```python
from build123d import *

# Parameters (mm, degrees)
F0_R     = 63.5
F1_DEPTH = 127
F2_R     = 25.4
F2_R_2   = 24.093414
F3_DEPTH = 127


with BuildPart() as f1:
    # F0 (on Front) → F1 (new body)
    with BuildSketch(Plane.XZ):
        with Locations((-63.626207, 65.614522)):
            Circle(F0_R)
    extrude(amount=F1_DEPTH)

    # F2 (on face) → F3 (join)
    with BuildSketch(Plane(origin=(0, 0, 0), x_dir=(-1, 0, 0), z_dir=(0, 1, 0))):
        with Locations((61.020497, 71.783684)):
            Circle(F2_R)
        with Locations((61.020497, 71.783684)):
            Circle(F2_R_2, mode=Mode.SUBTRACT)
    extrude(amount=F3_DEPTH)


solid = f1.part
```
CAD build for the part. Positions are in the model's coordinates, mm. A direction names the side the tool comes from. Round coordinates to 2 decimals unless told otherwise and drop trailing zeros. Order: outer loops, then holes, each group sorted by start corner. A loop starts at its lowest first (then second) coordinate and runs counter-clockwise, first axis right, second up.
Q1. Wall check: L1, parallel to Y at x = -28, z = 102.5; L2, parallel to X at y = 62.5, z = 86; L3, parallel to X at y = 71, z = 58.5. Give the ranges that are in metal, low to high.
Q2. Drop flat-ended pins along their axis: pin 1 (1.5 mm diameter, centred on x = -108, z = 104, fed in from +Y); pin 2 (1 mm diameter, centred on y = -97.5, z = 19.5, fed in from -X); pin 3 (6 mm diameter, centred on y = -47.5, z = 48, fed in from -X). Give the stop position or say it passes through.
Q3. Two-plate mould, pull along X, no slides. Class faces 1 (the flat face through (-79, 0, 52)), 2 (the cylindrical face through (-72.14, 62.61, 50.41)), 3 (the cylindrical face through (-77.392, -62.611, 3.625)): pulls with the +X half, pulls with the -X half, needs draft (parallel to the pull), parting line crosses it, or undercut.
Q4. Slice it at B-B (x = -100). Write the cut outline in (y, z), and give its area (3 significant figures).
Q5. Slice it at D-D (z = 54.5). Write the cut outline in (x, y), and give its area (3 significant figures).
Q6. Slice it at C-C (y = 69.5). Write the cut outline in (x, z).
Q7. Which spindle directions (+Z, -Z, +X, -X, +Y, -Y) get a long thin tool onto all of the face, cutting with end or side? Do faces 4 (the flat face through (-65, -127, 67)), 5 (the cylindrical face through (-40.864, 62.611, 56.328)). Say none if no direction does.
Q8. Slice it at A-A (z = 91). Write the cut outline in (x, y).
Results below:
1. L1: y = -127 to 0
1. L2: x = -82.07 to -80.47, -41.57 to -39.97
1. L3: x = -82.67 to -81.12, -40.92 to -39.37
2. pin 1: stops at y = 0
2. pin 2: stops at x = -107.8
2. pin 3: stops at x = -125.42
3. face 1: needs draft
3. face 2: undercut
3. face 3: parting line crosses it
4. outline: (-127, 13.56) - (0, 13.56) - (0, 117.66) - (-127, 117.66) - close
4. area: 13,200 mm2
5. outline: (-126.15, -127) - (-1.11, -127) - (-1.11, 0) - (-42.41, 0) - (-42.41, 127) - (-44.23, 127) - (-44.23, 0) - (-77.81, 0) - (-77.81, 127) - (-79.63, 127) - (-79.63, 0) - (-126.15, 0) - close
5. area: 16,300 mm2
6. outline: circle Ø50.8 at (-61.02, 71.78); hole circle Ø48.19 at (-61.02, 71.78)
7. face 4: +Z, -Z, +X, -X, -Y
7. face 5: +Y
8. outline: (-121.83, -127) - (-5.42, -127) - (-5.42, 0) - (-44.41, 0) - (-44.41, 127) - (-46.49, 127) - (-46.49, 0) - (-75.55, 0) - (-75.55, 127) - (-77.63, 127) - (-77.63, 0) - (-121.83, 0) - close
